from build123d import *

# Parameters (mm, degrees)
EXTRUDE_1_DEPTH     = 10
CUT_EXTRUDE_4_DEPTH = 85
SKETCH_6_R          = 1.5
CUT_EXTRUDE_5_DEPTH = 12.024906083
SKETCH_7_R          = 3.25
CUT_EXTRUDE_6_DEPTH = 8.024906083
SKETCH_8_R          = 8
EXTRUDE_2_DEPTH     = 30
SKETCH_9_R          = 3.5
CUT_EXTRUDE_7_DEPTH = 30
SKETCH_10_R         = 5.25
CUT_EXTRUDE_8_DEPTH = 24


with BuildPart() as part:
    # 草图1 → 凸台-拉伸1 (new body)
    with BuildSketch(Plane(origin=(0, 0, 0), x_dir=(1, 0, 0), z_dir=(0, 1, 0))):
        Polygon((-42, 5.5), (-42, 10.5), (42, 10.5), (42, 5.5), (42, -5.5), (31, -5.5), (31, 5.5), (-31, 5.5), (-31, -5.5), (-42, -5.5), align=None)
    extrude(amount=EXTRUDE_1_DEPTH)

    # 草图5 → 切除-拉伸4 (cut, through all)
    with BuildSketch(Plane.ZY.offset(42)):
        Polygon((-5.5, 10), (5.5, 6.636962504), (5.5, 10), align=None)
    extrude(amount=-CUT_EXTRUDE_4_DEPTH, mode=Mode.SUBTRACT)

    # 草图6 → 切除-拉伸5 (cut, through all)
    with BuildSketch(Plane(origin=(0, 12.692999356, -14.308403996), x_dir=(1, 0, 0), z_dir=(0, -0.956304756, -0.292371705))):
        with Locations((-36.5, 14.962180107)):
            Circle(SKETCH_6_R)
        with Locations((36.5, 14.962180107)):
            Circle(SKETCH_6_R)
    extrude(amount=CUT_EXTRUDE_5_DEPTH, mode=Mode.SUBTRACT)

    # 草图7 → 切除-拉伸6 (cut, through all)
    with BuildSketch(Plane(origin=(0, 3.782188354, 1.156331023), x_dir=(1, 0, 0), z_dir=(0, 0.956304756, 0.292371705))):
        with Locations((36.5, 2.432088544)):
            Circle(SKETCH_7_R)
        with Locations((-36.5, 2.432088544)):
            Circle(SKETCH_7_R)
    extrude(amount=-CUT_EXTRUDE_6_DEPTH, mode=Mode.SUBTRACT)

    # 草图8 → 凸台-拉伸2 (add)
    with BuildSketch(Plane.XZ):
        with Locations((0, -13.5)):
            Circle(SKETCH_8_R)
    extrude(amount=-EXTRUDE_2_DEPTH)

    # 草图9 → 切除-拉伸7 (cut)
    with BuildSketch(Plane(origin=(0, 30, 0), x_dir=(1, 0, 0), z_dir=(0, 1, 0))):
        with Locations((0, 13.5)):
            Circle(SKETCH_9_R)
    extrude(amount=-CUT_EXTRUDE_7_DEPTH, mode=Mode.SUBTRACT)

    # 草图10 → 切除-拉伸8 (cut)
    with BuildSketch(Plane.XZ):
        with Locations((0, -13.5)):
            Circle(SKETCH_10_R)
    extrude(amount=-CUT_EXTRUDE_8_DEPTH, mode=Mode.SUBTRACT)


solid = part.part
Verification items for the finished model (mm, model axes). A direction names the side the tool comes from. Give positions to 0.01 mm unless a question says otherwise; leave off trailing zeros. Write each loop counter-clockwise with the first axis right and the second up, starting at its lowest first coordinate (ties: lowest second). Pieces come first, ordered by that corner, then holes. Notation, with made-up numbers: (44.5, -27.75) - (97.5, -27.75) arc R10 cw to (97.5, -19.75) - close; hole circle Ø2 at (-38.75, 62.5). An arc over 180 degrees is marked (long way). Answer as CSV lines item,"result". Start each with the question number.
1. Sectioned sample at C-C (x = 32). Record the boundary of the cut face in (y, z).
2. Sectioned sample at A-A (z = -13.5). Record the boundary of the cut face in (x, y).
3. Sectioned sample at D-D (z = 3.5). Record the boundary of the cut face in (x, y).
4. Draft check along Y on faces 1 (the face through (-1.73, 14.79, -21.31)), 2 (the face through (-36.92, 3.35, -4.89)), 3 (the face through (-35.355, 8.716, -1.299)). Enter one of: pulls with the +Y half, pulls with the -Y half, needs draft (parallel to the pull), parting line crosses it, or undercut.
5. Set-up check for faces 4 (the face through (-4, 24, -13)), 5 (the face through (31, 4, 0)), 6 (the face through (36.08, 3.35, -4.89)): record each of +Z, -Z, +X, -X, +Y, -Y from which the full face is reachable in a straight line by a thin tool's end or side.
6. Depth check by flat-ended pin: pin 1 (12 mm diameter, centred on x = -14, z = -15, fed in from +Y); pin 2 (8 mm diameter, centred on x = -21, y = 3.5, fed in from -Z); pin 3 (11 mm diameter, centred on x = 0, y = 3.5, fed in from +Z). Enter the tip coordinate at first touch or a pass-through.
7. Sectioned sample at B-B (y = 16). Record the boundary of the cut face in (x, z).
8. Thickness scan on line 1 (Z direction, x = 0, y = 11.25); line 2 (X direction, y = 25.2, z = -13.5); line 3 (Z direction, x = 0, y = 26.75). Record the ranges inside material, lowest first.
Derived:
1,outline,"(0, -10.5) - (10, -10.5) - (10, -5.5) - (6.64, 5.5) - (0, 5.5) - close"
2,outline,"(-8, 0) - (-5.25, 0) - (-5.25, 24) - (-3.5, 24) - (-3.5, 30) - (-8, 30) - close; (3.5, 24) - (5.25, 24) - (5.25, 0) - (8, 0) - (8, 30) - (3.5, 30) - close"
3,outline,"(-42, 0) - (-31, 0) - (-31, 7.25) - (-42, 7.25) - close; (31, 0) - (42, 0) - (42, 7.25) - (31, 7.25) - close"
4,face 1,"needs draft"
4,face 2,"undercut"
4,face 3,"pulls with the +Y half"
5,face 4,"-Y"
5,face 5,"+Z, +Y, -Y"
5,face 6,"none"
6,pin 1,"y = 10"
6,pin 2,"z = -10.5"
6,pin 3,"z = -5.5"
7,outline,"circle Ø16 at (0, -13.5); hole circle Ø10.5 at (0, -13.5)"
8,line 1,"-21.5 to -18.75, -8.25 to -5.5"
8,line 2,"-8 to -3.5, 3.5 to 8"
8,line 3,"-21.5 to -17, -10 to -5.5"
